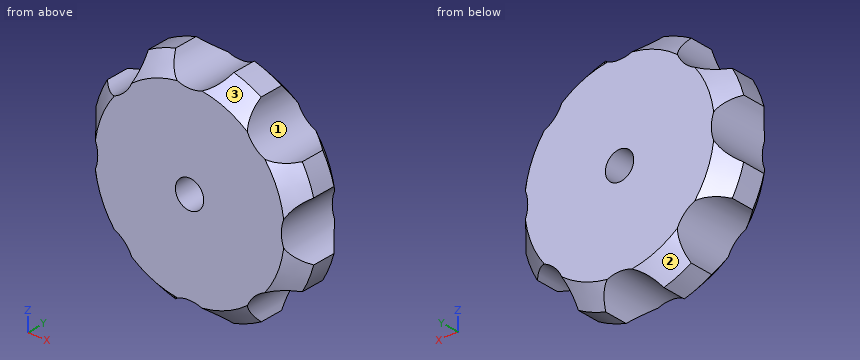
```python
from build123d import *

# Parameters (mm, degrees)
BOSS_EXTRUDE1_DEPTH  = 10
CHAMFER1_SIZE        = 3
M4_CLEARANCE_HOLE1_D = 4.8


with BuildPart() as part:
    # Sketch1 → Boss-Extrude1 (new body)
    with BuildSketch(Plane(origin=(0, 0, 0), x_dir=(1, 0, 0), z_dir=(0, 1, 0))):
        with BuildLine():
            ThreePointArc((4.929173178, -18.444040543), (0, -15.55551692), (-4.929173178, -18.444040543))
            ThreePointArc((-4.929173178, -18.444040543), (-7.30594069, -17.6381011), (-9.556454361, -16.527357921))
            ThreePointArc((-9.556454361, -16.527357921), (-10.999411499, -10.999411499), (-16.527357921, -9.556454361))
            ThreePointArc((-16.527357921, -9.556454361), (-17.6381011, -7.30594069), (-18.444040543, -4.929173178))
            ThreePointArc((-18.444040543, -4.929173178), (-15.55551692, 0), (-18.444040543, 4.929173178))
            ThreePointArc((-18.444040543, 4.929173178), (-17.6381011, 7.30594069), (-16.527357921, 9.556454361))
            ThreePointArc((-16.527357921, 9.556454361), (-10.999411499, 10.999411499), (-9.556454361, 16.527357921))
            ThreePointArc((-9.556454361, 16.527357921), (-7.30594069, 17.6381011), (-4.929173178, 18.444040543))
            ThreePointArc((-4.929173178, 18.444040543), (0, 15.55551692), (4.929173178, 18.444040543))
            ThreePointArc((4.929173178, 18.444040543), (7.30594069, 17.6381011), (9.556454361, 16.527357921))
            ThreePointArc((9.556454361, 16.527357921), (10.999411499, 10.999411499), (16.527357921, 9.556454361))
            ThreePointArc((16.527357921, 9.556454361), (17.6381011, 7.30594069), (18.444040543, 4.929173178))
            ThreePointArc((18.444040543, 4.929173178), (15.55551692, 0), (18.444040543, -4.929173178))
            ThreePointArc((18.444040543, -4.929173178), (17.6381011, -7.30594069), (16.527357921, -9.556454361))
            ThreePointArc((16.527357921, -9.556454361), (10.999411499, -10.999411499), (9.556454361, -16.527357921))
            ThreePointArc((9.556454361, -16.527357921), (7.30594069, -17.6381011), (4.929173178, -18.444040543))
        make_face()
    extrude(amount=BOSS_EXTRUDE1_DEPTH)

    # Chamfer1
    chamfer1_edges = [part.edges().sort_by_distance(p)[0] for p in [
        (7.30594069, 10, -17.6381011),
        (17.6381011, 0, 7.30594069),
        (7.30594069, 0, 17.6381011),
        (-7.30594069, 0, 17.6381011),
        (-17.6381011, 0, 7.30594069),
        (-17.6381011, 0, -7.30594069),
        (-7.30594069, 0, -17.6381011),
        (-7.30594069, 10, -17.6381011),
        (7.30594069, 0, -17.6381011),
        (17.6381011, 0, -7.30594069),
        (-17.6381011, 10, -7.30594069),
        (-17.6381011, 10, 7.30594069),
        (-7.30594069, 10, 17.6381011),
        (17.6381011, 10, -7.30594069),
        (7.30594069, 10, 17.6381011),
        (17.6381011, 10, 7.30594069),
    ]]
    chamfer(chamfer1_edges, length=CHAMFER1_SIZE)

    # M4 Clearance Hole1 (through all)
    with Locations(Plane(origin=(0, 10, 0), x_dir=(1, 0, 0), z_dir=(0, 1, 0))):
        with Locations((0, 0)):
            Hole(M4_CLEARANCE_HOLE1_D / 2)


solid = part.part
```
Geometry check sheet. Reference: the model listing, model coordinates, mm. Face numbers are marked on the shaded views. Coordinates: 2 decimals unless noted, no trailing zeros. Order: outer loops, then holes, each group sorted by start corner. A loop starts at its lowest first (then second) coordinate and runs counter-clockwise, first axis right, second up.
Item 1: Depth check by flat-ended pin: pin 1 (1 mm diameter, centred on x = 1, y = 8, fed in from +Z); pin 2 (6 mm diameter, centred on y = 8.5, z = -4.5, fed in from +X); pin 3 (4 mm diameter, centred on x = 14, y = 4, fed in from +Z); pin 4 (4 mm diameter, centred on x = -0.5, y = 6.5, fed in from -Z). Enter the tip coordinate at first touch or a pass-through.
Item 2: Section check A-A (x = 0). Enter the section's corners in (y, z), plus the area to 3 significant figures.
Item 3: Scan lines: line 1 along Z through (x, y) = (15, 2.25); line 2 along Z through (x, y) = (-2, 5.25); line 3 along Z through (x, y) = (6, 9). Record each from-to range of solid material in increasing order.
Item 4: Mould release check, pull along Z, two halves, no side actions. Record for the marked faces 1, 2 and 3: released by +Z, released by -Z, zero draft, split by the parting line, or undercut.
Item 5: Section check B-B (z = 0). Enter the section's corners in (x, y).
Item 6: Section check C-C (y = 7.5). Enter the section's corners in (x, z).
Item 7: Section check D-D (x = 10.5). Enter the section's corners in (y, z).
Check sheet entries:
1. pin 1: stops at z = 15.76
1. pin 2: stops at x = 18.44
1. pin 3: stops at z = 10.2
1. pin 4: stops at z = -16.14
2. outline: (0, -15.56) - (10, -15.56) - (10, -2.4) - (0, -2.4) - close; (0, 2.4) - (10, 2.4) - (10, 15.56) - (0, 15.56) - close
2. area: 263 mm2
3. line 1: z = -9.34 to 9.34
3. line 2: z = -15.92 to -1.33, 1.33 to 15.92
3. line 3: z = -16 to 16
4. face 1: undercut
4. face 2: released by -Z
4. face 3: released by +Z
5. outline: (-15.56, 0) - (-2.4, 0) - (-2.4, 10) - (-15.56, 10) - close; (2.4, 0) - (15.56, 0) - (15.56, 10) - (2.4, 10) - close
6. outline: (-18, -4.65) arc R18.59 ccw to (-16.02, -9.44) arc R5.65 cw to (-9.44, -16.02) arc R18.59 ccw to (-4.65, -18) arc R5.65 cw to (4.65, -18) arc R18.59 ccw to (9.44, -16.02) arc R5.65 cw to (16.02, -9.44) arc R18.59 ccw to (18, -4.65) arc R5.65 cw to (18, 4.65) arc R18.59 ccw to (16.02, 9.44) arc R5.65 cw to (9.44, 16.02) arc R18.59 ccw to (4.65, 18) arc R5.65 cw to (-4.65, 18) arc R18.59 ccw to (-9.44, 16.02) arc R5.65 cw to (-16.02, 9.44) arc R18.59 ccw to (-18, 4.65) arc R5.65 cw to start; hole circle Ø4.8 at (0, 0)
7. outline: (0, -11.57) - (10, -11.57) - (10, 11.57) - (0, 11.57) - close
